Design review of the part shown in the three views and the two pictorial views. Dimensions are in mm from the part's minimum x, y and z. A direction names the side the tool comes from. Round coordinates to 2 decimals unless told otherwise and drop trailing zeros. Order: outer loops, then holes, each group sorted by start corner. A loop starts at its lowest first (then second) coordinate and runs counter-clockwise, first axis right, second up. Notation, with made-up numbers: (0.25, 4.5) -> (55.25, 4.5) arc R21 cw to (55.25, 26.5) -> close; hole circle Ø2 at (-21, -17.75). An arc over 180 degrees is marked (long way). Put each result on its own line as item: value. Start each with the question number.
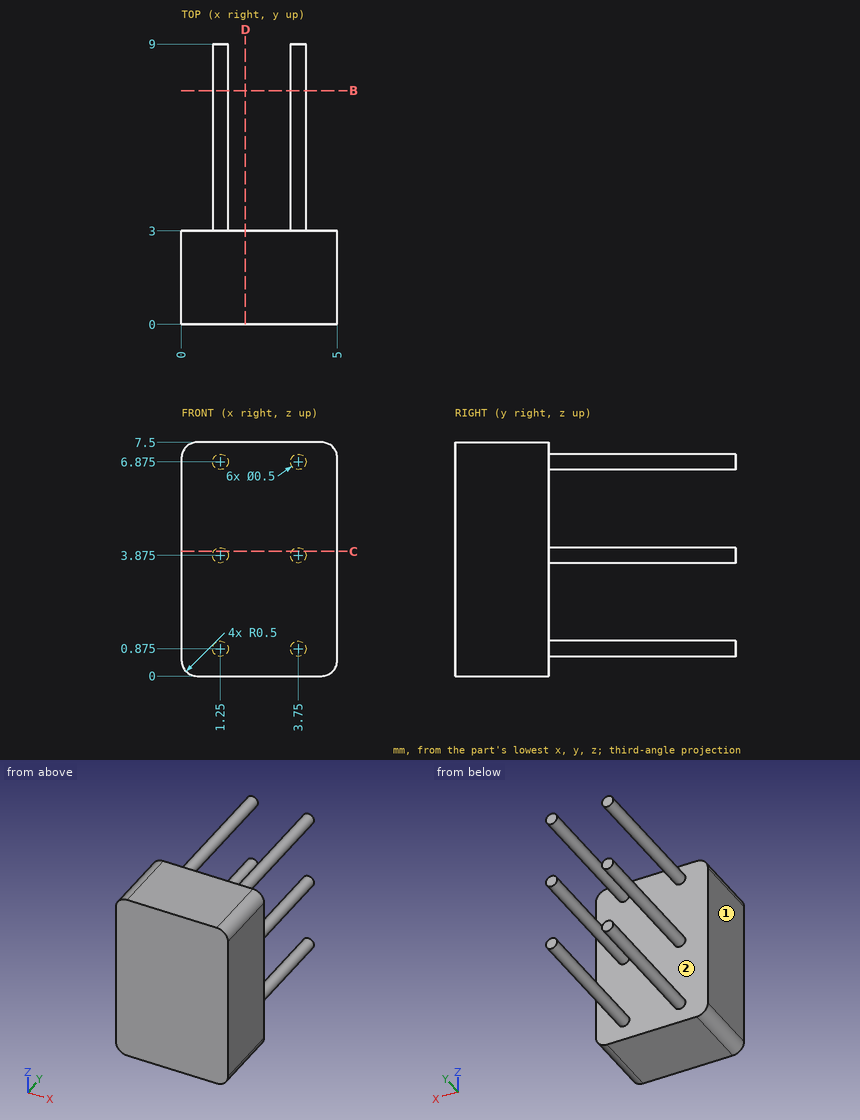
Q1. Wall thickness on probe 1 along Z at (x, y) = (1.1, 4) (1 decimal); probe 2 along Y at (x, z) = (3.95, 6.5); probe 3 along Z at (x, y) = (3.85, 8) (1 decimal): over which ranges is each line inside the solid? List them lowest first. Write a range as [from, to].
Q2. Take a section at D-D on x = 2.05. Give the boundary of the cut face in (y, z), and give its area (3 significant figures).
Q3. Take a section at C-C on z = 4. Give the boundary of the cut face in (x, y).
Q4. Clearance check with a flat-ended pin moving along its axis: pin 1 Ø1.5 at (y, z) = (7, 1) entering from +X. State where the tip first meets the part, or that it passes through.
Q5. For the marked faces 1 and 2, list the 3-axis set-ups (+Z, -Z, +X, -X, +Y, -Y) from which the entire face can be reached by the end or side of a thin tool; tool diameter is ignored.
Q6. Take a section at B-B on y = 7.5. State how many separate pieces and enclosed holes the cut face has.
Calculated:
1. probe 1: z = [0.7, 1.1], [3.7, 4.1], [6.7, 7.1]
1. probe 2: y = [0, 3]
1. probe 3: z = [0.6, 1.1], [3.6, 4.1], [6.6, 7.1]
2. outline: (0, 0) -> (3, 0) -> (3, 7.5) -> (0, 7.5) -> close
2. area: 22.5 mm²
3. outline: (0, 0) -> (5, 0) -> (5, 3) -> (3.97, 3) -> (3.97, 9) -> (3.53, 9) -> (3.53, 3) -> (1.47, 3) -> (1.47, 9) -> (1.03, 9) -> (1.03, 3) -> (0, 3) -> close
4. pin 1: stops at x = 4
5. face 1: +Z, -Z, -X, +Y, -Y
5. face 2: +Y
6. separate pieces: 6
6. enclosed holes: 0
